```python
from build123d import *

# Parameters (mm, degrees)
BOSS_EXTRUDE1_START = -9
SKETCH2_R           = 14
SKETCH2_W           = 9
SKETCH2_H           = 9
BOSS_EXTRUDE1_DEPTH = 5
BOSS_EXTRUDE2_START = -4
BOSS_EXTRUDE2_DEPTH = 4
CUT_EXTRUDE1_START  = 9
SKETCH4_W           = 25
SKETCH4_H           = 10
CUT_EXTRUDE1_DEPTH  = 13


with BuildPart() as part:
    # Sketch2 → Boss-Extrude1 (new body)
    with BuildSketch(Plane(origin=(0, 0, 0), x_dir=(0, 0, -1), z_dir=(1, 0, 0)).offset(BOSS_EXTRUDE1_START)):
        with BuildLine():
            Line((-20, 48), (-20, -252))
            Line((-20, -252), (20, -252))
            Line((20, -252), (20, 48))
            ThreePointArc((20, 48), (0, 68), (-20, 48))
        make_face()
        Circle(SKETCH2_R, mode=Mode.SUBTRACT)
        with Locations((0, 48)):
            Rectangle(SKETCH2_W, SKETCH2_H, mode=Mode.SUBTRACT)
    extrude(amount=BOSS_EXTRUDE1_DEPTH)

    # Sketch2<6> → Boss-Extrude2 (add)
    with BuildSketch(Plane(origin=(0, 0, 0), x_dir=(0, 0, -1), z_dir=(1, 0, 0)).offset(BOSS_EXTRUDE2_START)):
        with BuildLine():
            Line((-20, 48), (-20, -252))
            Line((-20, -252), (20, -252))
            Line((20, -252), (20, 48))
            ThreePointArc((20, 48), (0, 68), (-20, 48))
        make_face()
        with BuildLine():
            Line((15, 48), (15, -247))
            Line((15, -247), (-15, -247))
            Line((-15, -247), (-15, 48))
            ThreePointArc((-15, 48), (0, 63), (15, 48))
        make_face(mode=Mode.SUBTRACT)
    extrude(amount=BOSS_EXTRUDE2_DEPTH)

    # Mirror1: part across plane


with BuildPart() as part_1:
    add(part.part)
    add(part.part.mirror(Plane(origin=(0, 0, 0), x_dir=(0, 0, 1), z_dir=(1, 0, 0))))

    # Sketch4 → Cut-Extrude1 (cut)
    with BuildSketch(Plane(origin=(0, 0, 0), x_dir=(0, 0, -1), z_dir=(1, 0, 0)).offset(CUT_EXTRUDE1_START)):
        with Locations((0, -100)):
            Rectangle(SKETCH4_W, SKETCH4_H)
    extrude(amount=-CUT_EXTRUDE1_DEPTH, mode=Mode.SUBTRACT)


solid = part_1.part
```
Read the model definition and answer for the solid it produces. Units are mm, in the model's axes. A direction names the side the tool comes from. Give positions to 0.01 mm unless a question says otherwise; leave off trailing zeros. Order: outer loops, then holes, each group sorted by start corner. A loop starts at its lowest first (then second) coordinate and runs counter-clockwise, first axis right, second up.
(1) For a pull along Y with two mould halves and no side action, classify faces 6 (the flat face through (0, -104, -20)), 7 (the cylindrical face through (6.535, -5.362, -12.932)) as released by +Y, released by -Y, zero draft, split by the parting line, or undercut.
(2) Find section C-C (y = -184). Give the vertices of the cut face in (x, z), plus the area to 3 significant figures.
(3) Given pin 1 (4 mm diameter, centred on x = -6, z = 1.5, fed in from +Y); pin 2 (17 mm diameter, centred on y = 0, z = 0, fed in from +X); pin 3 (2.5 mm diameter, centred on x = 6, z = -5.5, fed in from +Y), each flat-ended and moving along its own axis, determine where each tip first touches the part or whether it passes through.
(4) Find section A-A (y = 0). Give the vertices of the cut face in (x, z).
(5) For faces 1 (the flat face through (-9, -90, 0)), 2 (the flat face through (0, -100, 20)), 3 (the flat face through (-7, 48, -4.5)), 4 (the flat face through (-4, -90, 0)), 5 (the flat face through (7, -95, 0)), determine the directions among +Z, -Z, +X, -X, +Y, -Y from which every point of the face is accessible in a straight line to the end or side of a thin tool.
(6) Find section B-B (z = 0). Give the vertices of the cut face in (x, y).
(7) Straight lines are drawn through the part: L1, parallel to Y at x = 5.65, z = 0; L2, parallel to Y at x = -6.8, z = 0; L3, parallel to X at y = -150.5, z = 12.5. For each, find the intervals that lie inside material, in ascending order.
Result sheet:
1. face 6: zero draft
1. face 7: undercut
2. outline: (-9, -20) - (9, -20) - (9, 20) - (-9, 20) - close; hole (-4, -15) - (4, -15) - (4, 15) - (-4, 15) - close
2. area: 480 mm2
3. pin 1: stops at y = 68
3. pin 2: passes through
3. pin 3: stops at y = 67.54
4. outline: (-9, -20) - (9, -20) - (9, -14) - (4, -14) - (4, -15) - (-4, -15) - (-4, -14) - (-9, -14) - close; (-9, 14) - (-4, 14) - (-4, 15) - (4, 15) - (4, 14) - (9, 14) - (9, 20) - (-9, 20) - close
5. face 1: +Z, -Z, -X, +Y, -Y
5. face 2: +Z, +X, -X, +Y, -Y
5. face 3: +X, -X
5. face 4: none
5. face 5: +X
6. outline: (-9, -252) - (9, -252) - (9, -105) - (4, -105) - (4, -247) - (-4, -247) - (-4, -14) - (-9, -14) - close; (-9, 14) - (-4, 14) - (-4, 43.5) - (-9, 43.5) - close; (-9, 52.5) - (-4, 52.5) - (-4, 63) - (4, 63) - (4, 52.5) - (9, 52.5) - (9, 68) - (-9, 68) - close; (4, -95) - (9, -95) - (9, -14) - (4, -14) - close; (4, 14) - (9, 14) - (9, 43.5) - (4, 43.5) - close
7. L1: y = -252 to -105, -95 to -14, 14 to 43.5, 52.5 to 68
7. L2: y = -252 to -14, 14 to 43.5, 52.5 to 68
7. L3: x = -9 to -4, 4 to 9
